Check sheet for the drawn part. Datum: minimum x, y, z corner. Units: mm. A direction names the side the tool comes from. Coordinates: 2 decimals unless noted, no trailing zeros. Loops run counter-clockwise (first coordinate to the right, second up) from the corner with the lowest first, then second, coordinate; pieces in that order, holes last. Notation, with made-up numbers: M 70.25,3 L 103.25,3 A10 ccw 103.25,16 Z; hole C -5,74 d3. An arc over 180 degrees is marked long. Answer as CSV lines item,"result". Start each with the question number.
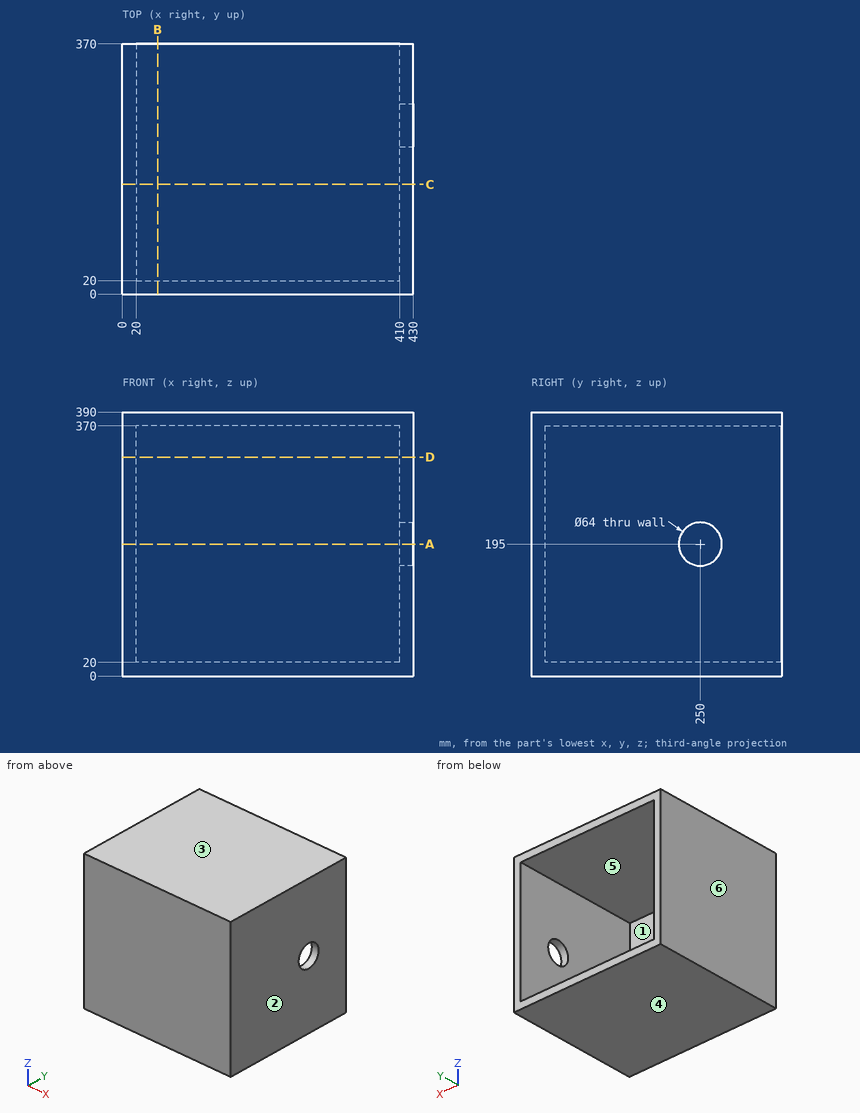
Item 1: Sectioned sample at D-D, the plane z = 323.5. Record the boundary of the cut face in (x, y).
Item 2: Go/stop test with a flat-tipped pin: pin 1 (1.5 mm diameter, centred on x = 111.5, z = 319, fed in from +Y). Record where the tip stops, or that it passes through.
Item 3: Release check for a two-part mould opening along Z. For the marked faces 3, 4, 5 and 6 record: released by +Z, released by -Z, zero draft, split by the parting line, or undercut.
Item 4: Sectioned sample at C-C, the plane y = 162.5. Record the boundary of the cut face in (x, z), and give its area (3 significant figures).
Item 5: Material ranges on line 1 (Z direction, x = 215, y = 148.5); line 2 (X direction, y = 276.5, z = 84); line 3 (Y direction, x = 424, z = 195), recorded low to high. Write a range as from..to.
Item 6: Sectioned sample at A-A, the plane z = 195. Record the boundary of the cut face in (x, y).
Item 7: Set-up check for the marked faces 1 and 2: record each of +Z, -Z, +X, -X, +Y, -Y from which the full face is reachable in a straight line by a thin tool's end or side.
Item 8: Sectioned sample at B-B, the plane x = 52. Record the boundary of the cut face in (y, z).
Reply:
1,outline,"M 0,0 L 430,0 L 430,370 L 410,370 L 410,20 L 20,20 L 20,370 L 0,370 Z"
2,pin 1,"y = 20"
3,face 3,"released by +Z"
3,face 4,"released by -Z"
3,face 5,"undercut"
3,face 6,"zero draft"
4,outline,"M 0,0 L 430,0 L 430,390 L 0,390 Z; hole M 20,20 L 410,20 L 410,370 L 20,370 Z"
4,area,"31,200 mm²"
5,line 1,"0..20, 370..390"
5,line 2,"0..20, 410..430"
5,line 3,"0..218, 282..370"
6,outline,"M 0,0 L 430,0 L 430,218 L 410,218 L 410,20 L 20,20 L 20,370 L 0,370 Z; M 410,282 L 430,282 L 430,370 L 410,370 Z"
7,face 1,"+Y"
7,face 2,"+Z, -Z, +X, +Y, -Y"
8,outline,"M 0,0 L 370,0 L 370,20 L 20,20 L 20,370 L 370,370 L 370,390 L 0,390 Z"
